Geometry check sheet. Reference: drawing and pictorial views, mm from the part's lowest x, y, z. A direction names the side the tool comes from. Give positions to 0.01 mm unless a question says otherwise; leave off trailing zeros. Loops run counter-clockwise (first coordinate to the right, second up) from the corner with the lowest first, then second, coordinate; pieces in that order, holes last. Notation, with made-up numbers: (-12, 6) - (44, 6) arc R25 ccw to (44, 19) - close; hole circle Ø5 at (5.25, -30). An arc over 180 degrees is marked (long way). Put each result on its own line as item: value. Start each with the question number.
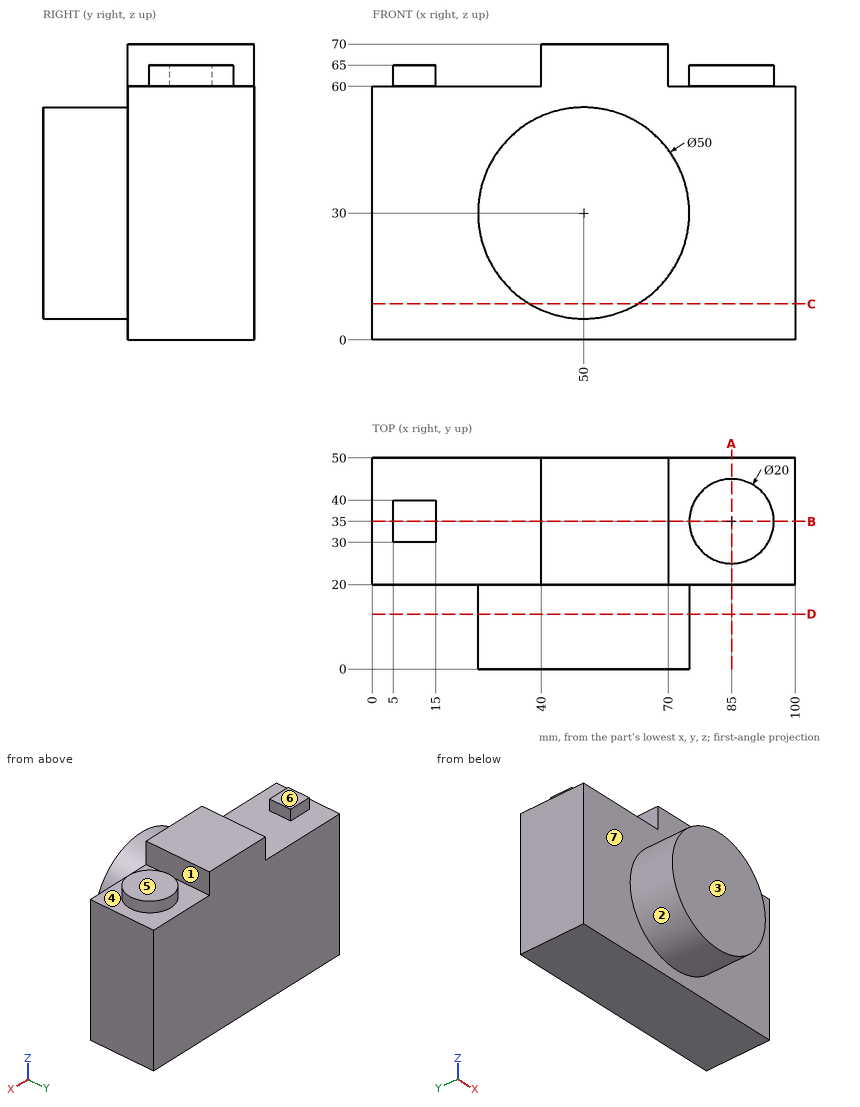
1) Section check D-D, the plane y = 13. Enter the section's corners in (x, z), plus the area to 3 significant figures.
2) Section check C-C, the plane z = 8.5. Enter the section's corners in (x, y), plus the area to 3 significant figures.
3) Scan lines: line 1 along X through (y, z) = (7, 29.5) (3 decimals); line 2 along Y through (x, z) = (93, 27.5); line 3 along X through (y, z) = (5, 15). Record each from-to range of solid material in increasing order. Write a range as from..to.
4) Set-up check for the marked faces 5, 6 and 7: record each of +Z, -Z, +X, -X, +Y, -Y from which the full face is reachable in a straight line by a thin tool's end or side.
5) Section check A-A, the plane x = 85. Enter the section's corners in (y, z).
6) Section check B-B, the plane y = 35. Enter the section's corners in (x, z), plus the area to 3 significant figures.
7) Depth check by flat-ended pin: P1, Ø4, axis at x = 12, z = 63.5, coming from the +Y side; P2, Ø6, axis at x = 82, y = 38.5, coming from the +Z side; P3, Ø8, axis at y = 11, z = 37, coming from the -X side. Enter the tip coordinate at first touch or a pass-through.
8) Draft check along X on the marked faces 1, 2, 3 and 4. Enter one of: pulls with the +X half, pulls with the -X half, needs draft (parallel to the pull), parting line crosses it, or undercut.
Results are:
1. outline: circle Ø50 at (50, 30)
1. area: 1,960 mm2
2. outline: (0, 20) - (37.24, 20) - (37.24, 0) - (62.76, 0) - (62.76, 20) - (100, 20) - (100, 50) - (0, 50) - close
2. area: 3,510 mm2
3. line 1: x = 25.005..74.995
3. line 2: y = 20..50
3. line 3: x = 30..70
4. face 5: +Z, +X, +Y, -Y
4. face 6: +Z, -X, +Y, -Y
4. face 7: -Y
5. outline: (20, 0) - (50, 0) - (50, 60) - (45, 60) - (45, 65) - (25, 65) - (25, 60) - (20, 60) - close
6. outline: (0, 0) - (100, 0) - (100, 60) - (95, 60) - (95, 65) - (75, 65) - (75, 60) - (70, 60) - (70, 70) - (40, 70) - (40, 60) - (15, 60) - (15, 65) - (5, 65) - (5, 60) - (0, 60) - close
6. area: 6,450 mm2
7. P1: stops at y = 40
7. P2: stops at z = 65
7. P3: stops at x = 25.18
8. face 1: undercut
8. face 2: parting line crosses it
8. face 3: needs draft
8. face 4: undercut
